Geometry check sheet. Reference: the model listing, model coordinates, mm. A direction names the side the tool comes from. Give positions to 0.01 mm unless a question says otherwise; leave off trailing zeros. Order: outer loops, then holes, each group sorted by start corner. A loop starts at its lowest first (then second) coordinate and runs counter-clockwise, first axis right, second up. Notation, with made-up numbers: M -20.75,-8.75 L -8.75,-8.75 A11 ccw -8.75,12.25 Z; hole C -12.5,-40 d4. An arc over 180 degrees is marked long. Use CSV: the item, a comma, the result in double quotes. Start each with the question number.
from build123d import *

# Parameters (mm, degrees)
F0_W     = 101.6
F0_H     = 50.8
F1_DEPTH = 25.4
F2_W     = 50.8
F2_H     = 12.7
F3_DEPTH = 25.401
F4_W     = 19.05
F4_H     = 12.7
F5_DEPTH = 25.401
F6_R     = 6.14583
F7_DEPTH = 50.8
F8_DEPTH = 50.801


with BuildPart() as f1:
    # F0 (on Front) → F1 (new body)
    with BuildSketch(Plane.XZ):
        Rectangle(F0_W, F0_H)
    extrude(amount=F1_DEPTH)

    # F2 (on Front) → F3 (cut, through all)
    with BuildSketch(Plane.XZ):
        with Locations((0, 19.05)):
            Rectangle(F2_W, F2_H)
    extrude(amount=F3_DEPTH, mode=Mode.SUBTRACT)

    # F4 (on Front) → F5 (cut, through all)
    with BuildSketch(Plane.XZ):
        with Locations((41.275, -19.05)):
            Rectangle(F4_W, F4_H)
    extrude(amount=F5_DEPTH, mode=Mode.SUBTRACT)

    # F6 (on Right) → F7 (cut)
    with BuildSketch(Plane.YZ):
        with Locations((-12.7, 5.715)):
            Circle(F6_R)
    extrude(amount=-F7_DEPTH, mode=Mode.SUBTRACT)

    # F6 (on Right) → F8 (cut, through all)
    with BuildSketch(Plane.YZ):
        with Locations((-12.7, 5.715)):
            Circle(F6_R)
    extrude(amount=F8_DEPTH, mode=Mode.SUBTRACT)


solid = f1.part
(1) Sectioned sample at B-B on y = -12.7. Record the cut outline in (x, z).
(2) Sectioned sample at A-A on z = 18.5. Record the cut outline in (x, y).
(3) Sectioned sample at C-C on y = -4.75. Record the cut outline in (x, z).
(4) Go/stop test with a flat-tipped pin: P1, Ø6.5, axis at y = -8, z = -21, coming from the +X side. Record where the tip stops, or that it passes through.
(5) Thickness scan on line 1 (X direction, y = -2, z = 21.5); line 2 (Z direction, x = 16, y = -12.7); line 3 (X direction, y = -21.75, z = -21.5). Record the ranges inside material, lowest first.
(6) Access from +Z, -Z, +X, -X, +Y, -Y to the whole of each face (thin tool, end or side, straight path). Record for faces 5 (the face through (25.4, -13, 19)), 6 (the face through (41, -13, -12.7)), 7 (the face through (50.8, -18, 2)).
(7) Sectioned sample at D-D on x = 28. Record the cut outline in (y, z) (3 decimals).
(8) Draft check along X on faces 1 (the face through (-1, 0, 0)), 2 (the face through (0, -13, 12.7)), 3 (the face through (31.75, -13, -19)), 4 (the face through (-50.8, -15.3, -0.4)). Enter one of: +X half, -X half, draft (parallel to the pull), parting line (faces both ways), or undercut.
Responses:
1,outline,"M -50.8,-25.4 L 31.75,-25.4 L 31.75,-12.7 L 50.8,-12.7 L 50.8,-0.43 L -50.8,-0.43 Z; M -50.8,11.86 L 50.8,11.86 L 50.8,25.4 L 25.4,25.4 L 25.4,12.7 L -25.4,12.7 L -25.4,25.4 L -50.8,25.4 Z"
2,outline,"M -50.8,-25.4 L -25.4,-25.4 L -25.4,0 L -50.8,0 Z; M 25.4,-25.4 L 50.8,-25.4 L 50.8,0 L 25.4,0 Z"
3,outline,"M -50.8,-25.4 L 31.75,-25.4 L 31.75,-12.7 L 50.8,-12.7 L 50.8,25.4 L 25.4,25.4 L 25.4,12.7 L -25.4,12.7 L -25.4,25.4 L -50.8,25.4 Z"
4,P1,"x = 31.75"
5,line 1,"-50.8 to -25.4, 25.4 to 50.8"
5,line 2,"-25.4 to -0.43, 11.86 to 12.7"
5,line 3,"-50.8 to 31.75"
6,face 5,"+Z, +Y, -Y"
6,face 6,"-Z, +X, +Y, -Y"
6,face 7,"+Z, -Z, +X, +Y, -Y"
7,outline,"M -25.4,-25.4 L 0,-25.4 L 0,25.4 L -25.4,25.4 Z; hole C -12.7,5.715 d12.292"
8,face 1,"draft"
8,face 2,"undercut"
8,face 3,"+X half"
8,face 4,"-X half"
